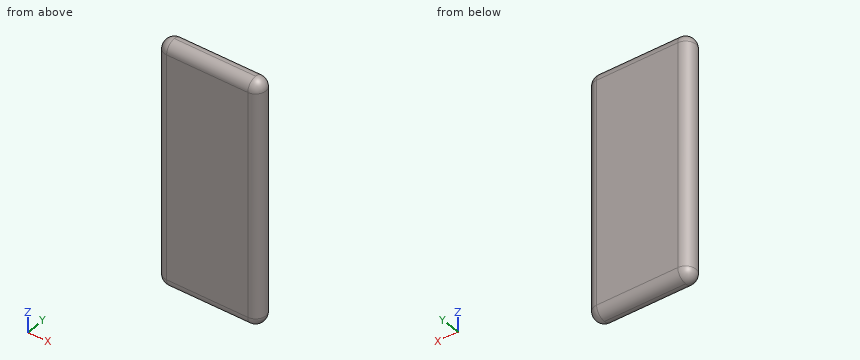
from build123d import *

# Parameters (mm, degrees)
BOSS_EXTRUDE1_DEPTH = 120
FILLET1_R           = 5


with BuildPart() as part:
    # Sketch1 → Boss-Extrude1 (new body)
    with BuildSketch(Plane.XY):
        with BuildLine():
            Line((0, 5), (40, 5))
            ThreePointArc((40, 5), (45, 0), (40, -5))
            Line((40, -5), (0, -5))
            ThreePointArc((0, -5), (-5, 0), (0, 5))
        make_face()
    extrude(amount=BOSS_EXTRUDE1_DEPTH)

    # Fillet1
    fillet1_edges = [part.edges().sort_by_distance(p)[0] for p in [
        (45, 0, 120),
        (20, 5, 120),
        (-5, 0, 120),
        (20, 5, 0),
        (45, 0, 0),
        (20, -5, 0),
        (-5, 0, 0),
        (20, -5, 120),
    ]]
    fillet(fillet1_edges, radius=FILLET1_R - 0.0001)  # a hair under: the kernel refuses the full size


solid = part.part
Verification items for the finished model (mm, model axes). Coordinates: 2 decimals unless noted, no trailing zeros. Order: outer loops, then holes, each group sorted by start corner. A loop starts at its lowest first (then second) coordinate and runs counter-clockwise, first axis right, second up. Notation, with made-up numbers: M -34.75,-36.75 L 1.25,-36.75 A21 cw 1.25,-1.75 Z; hole C 52,-7.5 d10. An arc over 180 degrees is marked long. One line per item, written item: value. Start each with the question number.
Item 1: Sectioned sample at B-B (z = 72). Enter the section's corners in (x, y), then the cut area to 3 significant figures.
Item 2: Gauge pin test, flat ends, axial feed: pin 1 (2 mm diameter, centred on x = 26.5, y = -3.5, fed in from +Z); pin 2 (4 mm diameter, centred on x = 28, y = -3, fed in from -Z). Record the tip position at first contact, or that the pin passes through.
Item 3: Scan lines: probe 1 along Z at (x, y) = (37.5, -0.25); probe 2 along X at (y, z) = (1.75, 24.5); probe 3 along Z at (x, y) = (-1.5, 1.75). Record each from-to range of solid material in increasing order.
Conclusion:
1. outline: M 0,-5 L 40,-5 A5 ccw 40,5 L 0,5 A5 ccw Z
1. area: 479 mm^2
2. pin 1: stops at z = 119.33
2. pin 2: stops at z = 0.1
3. probe 1: z = 0.01 to 119.99
3. probe 2: x = -4.68 to 44.68
3. probe 3: z = 0.56 to 119.44
